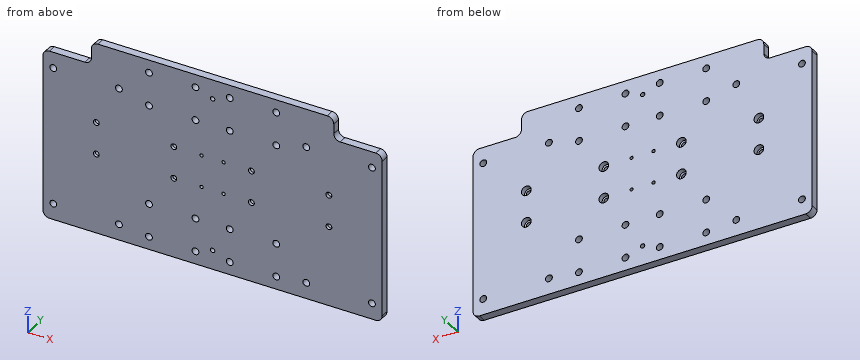
```python
from build123d import *

# Parameters (mm, degrees)
BOSS_EXTRUDE1_DEPTH            = 6.35
M10_CLEARANCE_HOLE1_D          = 10.5
CBORE_FOR_M8_SHCS1_D           = 9
CBORE_FOR_M8_SHCS1_CBORE_D     = 15
CBORE_FOR_M8_SHCS1_CBORE_DEPTH = 8
LPATTERN1_COUNT                = 2
LPATTERN1_PITCH                = 120
LPATTERN1_COL_COUNT            = 3
LPATTERN1_COL_PITCH            = 120
M6X1_0_TAPPED_HOLE1_D          = 5
M8X1_25_TAPPED_HOLE1_D         = 6.8


with BuildPart() as part:
    # Sketch1 → Boss-Extrude1 (new, symmetric)
    with BuildSketch(Plane(origin=(0, 0, 0), x_dir=(1, 0, 0), z_dir=(0, 1, 0))):
        with BuildLine():
            Line((-252.5, -115), (-197.5, -115))
            ThreePointArc((-197.5, -115), (-190.428932188, -117.928932188), (-187.5, -125))
            Line((-187.5, -125), (-187.5, -140))
            ThreePointArc((-187.5, -140), (-184.571067812, -147.071067812), (-177.5, -150))
            Line((-177.5, -150), (177.5, -150))
            ThreePointArc((177.5, -150), (184.571067812, -147.071067812), (187.5, -140))
            Line((187.5, -140), (187.5, -125))
            ThreePointArc((187.5, -125), (190.428932188, -117.928932188), (197.5, -115))
            Line((197.5, -115), (252.5, -115))
            ThreePointArc((252.5, -115), (259.571067812, -112.071067812), (262.5, -105))
            Line((262.5, -105), (262.5, 140))
            ThreePointArc((262.5, 140), (259.571067812, 147.071067812), (252.5, 150))
            Line((252.5, 150), (-252.5, 150))
            ThreePointArc((-252.5, 150), (-259.571067812, 147.071067812), (-262.5, 140))
            Line((-262.5, 140), (-262.5, -105))
            ThreePointArc((-262.5, -105), (-259.571067812, -112.071067812), (-252.5, -115))
        make_face()
    extrude(amount=BOSS_EXTRUDE1_DEPTH, both=True)

    # M10 Clearance Hole1 (through all)
    with Locations(Plane(origin=(0, 6.35, 0), x_dir=(1, 0, 0), z_dir=(0, 1, 0))):
        with Locations((-98.5, -130), (-26.5, -130), (-26.5, -78), (-98.5, -78), (98.5, -78), (26.5, -78), (26.5, -130), (98.5, -130), (98.5, 130), (26.5, 130), (26.5, 78), (98.5, 78), (-98.5, 78), (-26.5, 78), (-26.5, 130), (-98.5, 130), (-246.6, 125), (-145, 125), (-145, -90), (-246.6, -90), (145, -90), (246.6, -90), (145, 125), (246.6, 125)):
            Hole(M10_CLEARANCE_HOLE1_D / 2)

    # CBORE for M8 SHCS1 (through all)
    with Locations(Plane(origin=(0, 6.35, 0), x_dir=(1, 0, 0), z_dir=(0, 1, 0))):
        with Locations((60, 25), (60, -25)):
            cbore_for_m8_shcs1 = CounterBoreHole(CBORE_FOR_M8_SHCS1_D / 2, CBORE_FOR_M8_SHCS1_CBORE_D / 2, CBORE_FOR_M8_SHCS1_CBORE_DEPTH)

    # LPattern1: CBORE for M8 SHCS1 ×2
    with Locations(*[(i * LPATTERN1_PITCH, 0, 0) for i in range(1, LPATTERN1_COUNT)]):
        add(cbore_for_m8_shcs1, mode=Mode.SUBTRACT)

    # LPattern1 col: CBORE for M8 SHCS1 ×3
    with Locations(*[(-i * LPATTERN1_COL_PITCH, 0, 0) for i in range(1, LPATTERN1_COL_COUNT)]):
        add(cbore_for_m8_shcs1, mode=Mode.SUBTRACT)

    # M6x1.0 Tapped Hole1 (through all)
    with Locations(Plane(origin=(0, 6.35, 0), x_dir=(1, 0, 0), z_dir=(0, 1, 0))):
        with Locations((17, 25), (17, -25), (-17, -25), (-17, 25)):
            Hole(M6X1_0_TAPPED_HOLE1_D / 2)

    # M8x1.25 Tapped Hole1 (through all)
    with Locations(Plane(origin=(0, 6.35, 0), x_dir=(1, 0, 0), z_dir=(0, 1, 0))):
        with Locations((0, -120), (0, 120)):
            Hole(M8X1_25_TAPPED_HOLE1_D / 2)


solid = part.part
```
The model under review builds one solid part; all positions refer to its coordinate system, in mm. Give positions to 0.01 mm unless a question says otherwise; leave off trailing zeros. Write each loop counter-clockwise with the first axis right and the second up, starting at its lowest first coordinate (ties: lowest second). Pieces come first, ordered by that corner, then holes.
(1) For P1, Ø7.5, axis at x = -57, z = -23.5, coming from the +Y side; P2, Ø8.5, axis at x = -98.5, z = 130, coming from the +Y side, all flat-tipped, find the tip position at first contact; note any pin that passes through.
(2) Consider section C-C, the plane y = -4.25. Give the number of separate pieces and of enclosed holes in the cut face, and give its area (3 significant figures).
(3) To check wall thickness, follow L1, parallel to Z at x = 26.5, y = -1; L2, parallel to Z at x = 60, y = 0.75; L3, parallel to Z at x = -186, y = 1.25. State the ranges of each line that lie inside material, in increasing order.
(4) Consider section A-A, the plane x = 145. Give the boundary of the cut face in (y, z), and give its area (3 significant figures).
(5) Consider section B-B, the plane z = -78. Give the boundary of the cut face in (x, y).
Returned:
1. P1: stops at y = -1.65
1. P2: passes through
2. separate pieces: 1
2. enclosed holes: 38
2. area: 149,000 mm2
3. L1: z = -150 to -135.25, -124.75 to -83.25, -72.75 to 72.75, 83.25 to 124.75, 135.25 to 150
3. L2: z = -150 to -32.5, -17.5 to 17.5, 32.5 to 150
3. L3: z = -150 to -29.5, -20.5 to 20.5, 29.5 to 145.27
4. outline: (-6.35, -150) - (6.35, -150) - (6.35, -130.25) - (-6.35, -130.25) - close; (-6.35, -119.75) - (6.35, -119.75) - (6.35, 84.75) - (-6.35, 84.75) - close; (-6.35, 95.25) - (6.35, 95.25) - (6.35, 150) - (-6.35, 150) - close
4. area: 3,540 mm2
5. outline: (-262.5, -6.35) - (-103.75, -6.35) - (-103.75, 6.35) - (-262.5, 6.35) - close; (-93.25, -6.35) - (-31.75, -6.35) - (-31.75, 6.35) - (-93.25, 6.35) - close; (-21.25, -6.35) - (21.25, -6.35) - (21.25, 6.35) - (-21.25, 6.35) - close; (31.75, -6.35) - (93.25, -6.35) - (93.25, 6.35) - (31.75, 6.35) - close; (103.75, -6.35) - (262.5, -6.35) - (262.5, 6.35) - (103.75, 6.35) - close
